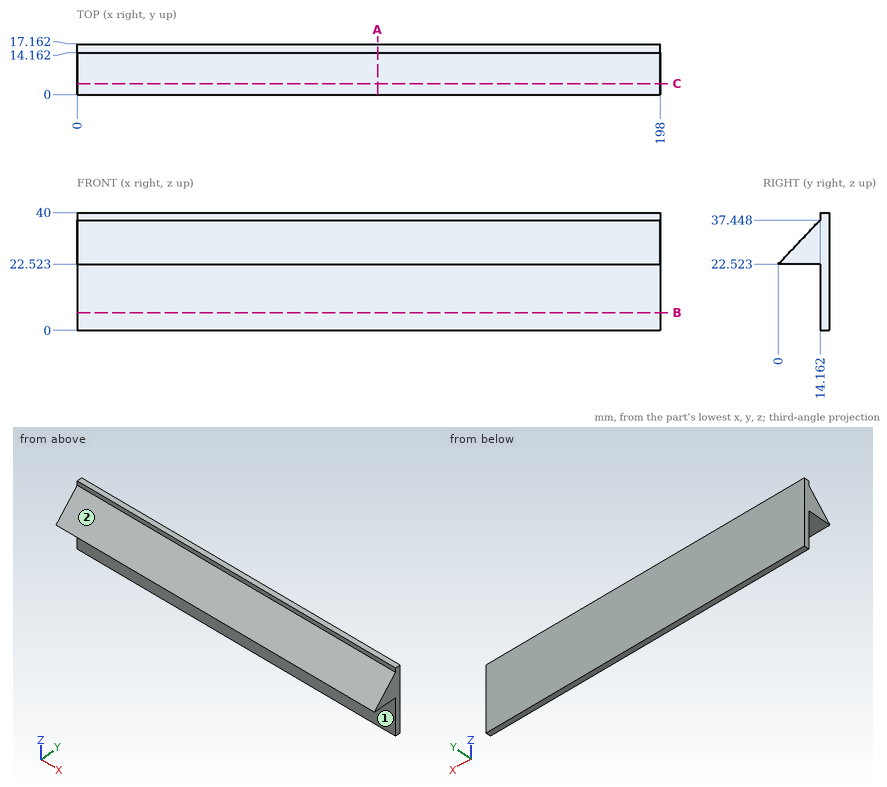
Source: three-view drawing plus pictorial views. Frame: mm from the lowest corner of the part. Coordinates: 2 decimals unless noted, no trailing zeros. Order: outer loops, then holes, each group sorted by start corner. A loop starts at its lowest first (then second) coordinate and runs counter-clockwise, first axis right, second up.
1) Draft query along Z for the marked faces 1 and 2. Return one class per face: released by +Z, released by -Z, zero draft, split by the parting line, or undercut.
Result sheet:
face 1: zero draft
face 2: released by +Z
2) Section C-C (y = 3.75). Return loops of the section in (x, z) (1 decimal).
Result sheet:
outline: (0, 22.5) - (198, 22.5) - (198, 26.5) - (0, 26.5) - close
3) Ray query, probe 1 along Y at (x, z) = (61, 37.5); probe 2 along Y at (x, z) = (173, 28) (1 decimal); probe 3 along Z at (x, y) = (30.5, 1.25) (1 decimal). Return the intervals inside material, ascending.
Result sheet:
probe 1: y = 14.16 to 17.16
probe 2: y = 5.2 to 17.2
probe 3: z = 22.5 to 23.8
4) Section A-A (x = 102). Return loops of the section in (y, z), then the cut area to 3 significant figures.
Result sheet:
outline: (0, 22.52) - (14.16, 22.52) - (14.16, 0) - (17.16, 0) - (17.16, 40) - (14.16, 40) - (14.16, 37.45) - close
area: 226 mm2
5) First-contact query: P1, Ø1.5, axis at x = 97, z = 12.5, coming from the -Y side; P2, Ø4, axis at x = 126, y = 9.5, coming from the +Z side; P3, Ø2, axis at x = 34.5, y = 6.5, coming from the +Z side. Flat tips, straight axial feed; report the tip coordinate or a pass-through.
Result sheet:
P1: stops at y = 14.16
P2: stops at z = 34.64
P3: stops at z = 30.43
6) Section B-B (z = 6). Return loops of the section in (x, y), then the cut area to 3 significant figures.
Result sheet:
outline: (0, 14.16) - (198, 14.16) - (198, 17.16) - (0, 17.16) - close
area: 594 mm2
